from build123d import *

# Parameters (mm, degrees)
SKETCH1_W           = 25
SKETCH1_H           = 25
BOSS_EXTRUDE1_DEPTH = 120
CUT_EXTRUDE1_DEPTH  = 120
SKETCH3_W           = 25
SKETCH3_H           = 12.5
CUT_EXTRUDE2_DEPTH  = 120
FILLET1_R           = 2.5
FILLET2_R           = 2.5
FILLET3_R           = 2.5
SKETCH6_R           = 2.75
CUT_EXTRUDE3_DEPTH  = 10
SKETCH7_W           = 10.05
SKETCH7_H           = 15.1
CUT_EXTRUDE4_DEPTH  = 2.5
SKETCH9_R           = 6.5
BOSS_EXTRUDE3_DEPTH = 7.5
BOSS_EXTRUDE3_DRAFT = -6
FILLET4_R           = 2.5
CHAMFER1_SIZE       = 1
CHAMFER1_SIZE2      = 0.909876415


with BuildPart() as part:
    # Sketch1 → Boss-Extrude1 (new body)
    with BuildSketch(Plane(origin=(0, 0, 0), x_dir=(1, 0, 0), z_dir=(0, 1, 0))):
        Rectangle(SKETCH1_W, SKETCH1_H)
    extrude(amount=BOSS_EXTRUDE1_DEPTH)

    # Sketch2 → Cut-Extrude1 (cut)
    with BuildSketch(Plane(origin=(0, 120, 0), x_dir=(1, 0, 0), z_dir=(0, 1, 0))):
        Polygon((-10.25, -2.48824277), (-10.25, -10.25), (-2.61175723, -10.25), (-2.61175723, -5.15), (2.48824277, -5.15), (2.48824277, -10.25), (10.25, -10.25), (10.25, -2.61175723), (5.15, -2.61175723), (5.15, 2.48824277), (10.25, 2.48824277), (10.25, 10.25), (2.61175723, 10.25), (2.61175723, 5.15), (-2.48824277, 5.15), (-2.48824277, 10.25), (-10.25, 10.25), (-10.25, 2.61175723), (-5.15, 2.61175723), (-5.15, -2.48824277), align=None)
    extrude(amount=-CUT_EXTRUDE1_DEPTH, mode=Mode.SUBTRACT)

    # Sketch3 → Cut-Extrude2 (cut)
    with BuildSketch(Plane(origin=(0, 120, 0), x_dir=(1, 0, 0), z_dir=(0, 1, 0))):
        with Locations((0, 6.25)):
            Rectangle(SKETCH3_W, SKETCH3_H)
    extrude(amount=-CUT_EXTRUDE2_DEPTH, mode=Mode.SUBTRACT)

    # Fillet1
    fillet1_edges = [part.edges().sort_by_distance(p)[0] for p in [
        (-12.5, 60, 0),
    ]]
    fillet(fillet1_edges, radius=FILLET1_R)

    # Fillet2
    fillet2_edges = [part.edges().sort_by_distance(p)[0] for p in [
        (12.5, 60, 0),
    ]]
    fillet(fillet2_edges, radius=FILLET2_R)

    # Fillet3
    # the kernel refuses this fillet: 2.5 mm, written as the material it takes off along each edge
    with BuildSketch(Plane(origin=(-10, 0, 0), x_dir=(0, 0, 1), z_dir=(1, 0, 0)), Plane(origin=(-1.1, 0, 0), x_dir=(0, 0, 1), z_dir=(1, 0, 0)), Plane(origin=(-10, 120, 0), x_dir=(0, -1, 0), z_dir=(1, 0, 0)), Plane(origin=(-1.1, 120, 0), x_dir=(0, -1, 0), z_dir=(1, 0, 0))) as fillet3_piece_1:
        with BuildLine():
            CenterArc((FILLET3_R, -FILLET3_R), FILLET3_R, 90, 90)
            Line((0, -FILLET3_R), (0, 0))
            Line((0, 0), (FILLET3_R, 0))
        make_face()
    extrude(amount=11.1, mode=Mode.SUBTRACT)
    with BuildSketch(Plane(origin=(-10, 0, 2.5), x_dir=(-1, 0, 0), z_dir=(0, 0, 1))) as fillet3_piece_2:
        with BuildLine():
            CenterArc((2.5 - FILLET3_R, -FILLET3_R), FILLET3_R, 0, 90)
            Line((2.5, -FILLET3_R), (2.5, 0))
            Line((2.5, 0), (2.5 - FILLET3_R, 0))
        make_face()
    revolve(axis=Axis((-10, 0, 2.5), (0, -1, 0)), revolution_arc=90, mode=Mode.SUBTRACT)
    with BuildSketch(Plane(origin=(10, 0, 2.5), x_dir=(1, 0, 0), z_dir=(0, 0, 1))) as fillet3_piece_3:
        with BuildLine():
            CenterArc((2.5 - FILLET3_R, FILLET3_R), FILLET3_R, 270, 90)
            Line((2.5, FILLET3_R), (2.5, 0))
            Line((2.5, 0), (2.5 - FILLET3_R, 0))
        make_face()
    revolve(axis=Axis((10, 0, 2.5), (0, 1, 0)), revolution_arc=90, mode=Mode.SUBTRACT)
    with BuildSketch(Plane(origin=(-10, 120, 2.5), x_dir=(-1, 0, 0), z_dir=(0, 0, 1))) as fillet3_piece_4:
        with BuildLine():
            CenterArc((2.5 - FILLET3_R, FILLET3_R), FILLET3_R, 270, 90)
            Line((2.5 - FILLET3_R, 0), (2.5, 0))
            Line((2.5, 0), (2.5, FILLET3_R))
        make_face()
    revolve(axis=Axis((-10, 120, 2.5), (0, -1, 0)), revolution_arc=90, mode=Mode.SUBTRACT)
    with BuildSketch(Plane(origin=(10, 120, 2.5), x_dir=(1, 0, 0), z_dir=(0, 0, 1))) as fillet3_piece_5:
        with BuildLine():
            CenterArc((2.5 - FILLET3_R, -FILLET3_R), FILLET3_R, 0, 90)
            Line((2.5 - FILLET3_R, 0), (2.5, 0))
            Line((2.5, 0), (2.5, -FILLET3_R))
        make_face()
    revolve(axis=Axis((10, 120, 2.5), (0, 1, 0)), revolution_arc=90, mode=Mode.SUBTRACT)
    with BuildSketch(Plane(origin=(-18.75, 0, 12.5), x_dir=(0, 0, -1), z_dir=(1, 0, 0)), Plane(origin=(-18.75, 120, 12.5), x_dir=(0, -1, 0), z_dir=(1, 0, 0))) as fillet3_piece_6:
        with BuildLine():
            CenterArc((FILLET3_R, FILLET3_R), FILLET3_R, 180, 90)
            Line((0, FILLET3_R), (0, 0))
            Line((0, 0), (FILLET3_R, 0))
        make_face()
    extrude(amount=37.5, mode=Mode.SUBTRACT)
    with BuildSketch(Plane(origin=(-12.5, 0, 2.5), x_dir=(1, 0, 0), z_dir=(0, 0, 1)), Plane(origin=(12.5, 0, 18.75), x_dir=(-1, 0, 0), z_dir=(0, 0, -1)), Plane(origin=(-12.5, 120, 2.5), x_dir=(0, -1, 0), z_dir=(0, 0, 1)), Plane(origin=(12.5, 120, 18.75), x_dir=(0, -1, 0), z_dir=(0, 0, -1))) as fillet3_piece_7:
        with BuildLine():
            CenterArc((FILLET3_R, FILLET3_R), FILLET3_R, 180, 90)
            Line((0, FILLET3_R), (0, 0))
            Line((0, 0), (FILLET3_R, 0))
        make_face()
    extrude(amount=16.25, mode=Mode.SUBTRACT)

    # Sketch6 → Cut-Extrude3 (cut)
    with BuildSketch(Plane.XY.offset(12.5)):
        with Locations((0, 107.5)):
            Circle(SKETCH6_R)
        with Locations((0, 12.5)):
            Circle(SKETCH6_R)
    extrude(amount=-CUT_EXTRUDE3_DEPTH, mode=Mode.SUBTRACT)

    # Sketch7 → Cut-Extrude4 (cut)
    with BuildSketch(Plane(origin=(0, 0, 5.15), x_dir=(-1, 0, 0), z_dir=(0, 0, -1))):
        with Locations((0, 107.5)):
            Rectangle(SKETCH7_W, SKETCH7_H)
        with Locations((0, 12.5)):
            Rectangle(SKETCH7_W, SKETCH7_H)
    extrude(amount=-CUT_EXTRUDE4_DEPTH, mode=Mode.SUBTRACT)


with BuildPart() as boss_extrude3_tool:
    # Sketch9 → Boss-Extrude3 (with draft: the straight prism first)
    with BuildSketch(Plane.XY.offset(20)):
        with Locations((0, 58.75)):
            Circle(SKETCH9_R)
    extrude(amount=-BOSS_EXTRUDE3_DEPTH)
    # Boss-Extrude3: the draft: its side faces are tilted about the plane it starts from
    boss_extrude3_sides = [boss_extrude3_tool.faces().sort_by_distance(p)[0] for p in [
        (-6.5, 58.75, 16.25),
    ]]
    draft(boss_extrude3_sides, Plane.XY.offset(20), BOSS_EXTRUDE3_DRAFT)


with BuildPart() as part_1:
    add(part.part)

    # Boss-Extrude3: add boss_extrude3_tool
    add(boss_extrude3_tool.part)

    # Fillet4
    fillet4_edges = [part_1.edges().sort_by_distance(p)[0] for p in [
        (-6.5, 58.75, 20),
    ]]
    fillet(fillet4_edges, radius=FILLET4_R)

    # Chamfer1
    chamfer1_edges = [part_1.edges().sort_by_distance(p)[0] for p in [
        (-5.711718236, 58.75, 12.5),
    ]]
    chamfer1_side = [part_1.faces().sort_by_distance(p)[0] for p in [
        (0, 3.67686023, 12.5),
    ]]
    chamfer(chamfer1_edges, length=CHAMFER1_SIZE, length2=CHAMFER1_SIZE2, reference=chamfer1_side[0])


solid = part_1.part
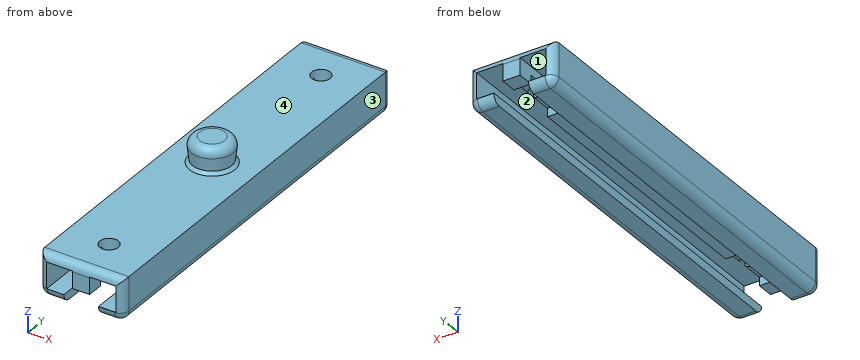
Here's how the part is built. I have some questions about the finished solid (model axes, mm). Face numbers are marked on the shaded views. Round coordinates to 2 decimals unless told otherwise and drop trailing zeros. Order: outer loops, then holes, each group sorted by start corner. A loop starts at its lowest first (then second) coordinate and runs counter-clockwise, first axis right, second up. Notation, with made-up numbers: M 29,43 L 56,43 A18 cw 56,64 Z; hole C 71,79 d2. An arc over 180 degrees is marked long. Return JSON: item names as keys, results as strings. Group by question number.
1. If we section it at B-B on y = 74: List the corners of the cut face in (x, z) for me, then the cut area to 3 significant figures.
2. Please list where these lines run through material, in increasing order: probe 1 along Y at (x, z) = (0, 9.7); probe 2 along X at (y, z) = (49, 5.5); probe 3 along Z at (x, y) = (-9, 11).
3. If we section it at A-A on x = 0: State how many separate pieces and enclosed holes the cut face has, then the cut area to 3 significant figures.
4. If we section it at C-C on y = 58.75: List the corners of the cut face in (x, z) for me, then the cut area to 3 significant figures.
5. If we mould it in two halves opening along Z, with no side actions, what happens to the marked faces 1, 2, 3 and 4? For each: pulls with the +Z half, pulls with the -Z half, needs draft (parallel to the pull), parting line crosses it, or undercut.
6. I'm going to push flat-ended pins straight in: pin 1 Ø10 at (x, z) = (8, 8) entering from -Y; pin 2 Ø3 at (x, z) = (3, 3) entering from +Y; pin 3 Ø1.5 at (x, z) = (0.5, 13) entering from +Y; pin 4 Ø4 at (x, y) = (7.5, 36) entering from +Z. Where does each tip first touch, or does it pass through?
Reply:
{
 "1": {"outline": "M -12.5,2.5 A2.5 ccw -10,0 L -5.15,0 L -5.15,2.49 L -10.25,2.49 L -10.25,10.25 L -2.61,10.25 L -2.61,5.15 L 2.49,5.15 L 2.49,10.25 L 10.25,10.25 L 10.25,2.61 L 5.15,2.61 L 5.15,0 L 10,0 A2.5 ccw 12.5,2.5 L 12.5,12.5 L -12.5,12.5 Z", "area": "152 mm^2"},
 "2": {"probe 1": "0 to 9.75, 15.25 to 104.75, 110.25 to 120", "probe 2": "-12.5 to -10.25, -2.61 to 2.49, 10.25 to 12.5", "probe 3": "0 to 2.49, 10.25 to 12.5"},
 "3": {"separate pieces": "3", "enclosed holes": "0", "area": "840 mm^2"},
 "4": {"outline": "M -12.5,2.5 A2.5 ccw -10,0 L -5.15,0 L -5.15,2.49 L -10.25,2.49 L -10.25,10.25 L -2.61,10.25 L -2.61,5.15 L 2.49,5.15 L 2.49,10.25 L 10.25,10.25 L 10.25,2.61 L 5.15,2.61 L 5.15,0 L 10,0 A2.5 ccw 12.5,2.5 L 12.5,12.5 L 6.71,12.5 L 5.81,13.4 L 6.21,17.24 A2.5 ccw 3.72,20 L -3.72,20 A2.5 ccw -6.21,17.24 L -5.81,13.4 L -6.71,12.5 L -12.5,12.5 Z", "area": "241 mm^2"},
 "5": {"face 1": "undercut", "face 2": "undercut", "face 3": "needs draft", "face 4": "pulls with the +Z half"},
 "6": {"pin 1": "y = 0.01", "pin 2": "through", "pin 3": "y = 118.59", "pin 4": "z = 12.5"}
}
